```python
from build123d import *

# Parameters (mm, degrees)
F1_DEPTH = 150
F2_SIZE  = 20


with BuildPart() as f1:
    # F0 (on Top) → F1 (new body)
    with BuildSketch(Plane.XY):
        with BuildLine():
            ThreePointArc((40, 13), (36.485281, 21.485281), (28, 25))
            Line((28, 25), (5, 25))
            Line((5, 25), (5, 15))
            Line((5, 15), (-5, 15))
            Line((-5, 15), (-5, 25))
            Line((-5, 25), (-40, 25))
            Line((-40, 25), (-40, -13))
            ThreePointArc((-40, -13), (-36.485281, -21.485281), (-28, -25))
            Line((-28, -25), (-5, -25))
            Line((-5, -25), (-5, -15))
            Line((-5, -15), (5, -15))
            Line((5, -15), (5, -25))
            Line((5, -25), (40, -25))
            Line((40, -25), (40, 13))
        make_face()
        with BuildLine():
            ThreePointArc((-18.122446, 8.968033), (-23.391993, 14.619996), (-16.00245, 12.360026))
            Line((-16.00245, 12.360026), (-3.737005, 4.694123))
            ThreePointArc((-3.737005, 4.694123), (3.179994, 5.08799), (5.857001, -1.30213))
            Line((5.857001, -1.30213), (18.122446, -8.968033))
            ThreePointArc((18.122446, -8.968033), (23.391993, -14.619996), (16.00245, -12.360026))
            Line((16.00245, -12.360026), (3.737005, -4.694123))
            ThreePointArc((3.737005, -4.694123), (-3.179994, -5.08799), (-5.857001, 1.30213))
            Line((-5.857001, 1.30213), (-18.122446, 8.968033))
        make_face(mode=Mode.SUBTRACT)
    extrude(amount=F1_DEPTH)

    # F2
    f2_edges = [f1.edges().sort_by_distance(p)[0] for p in [
        (-40, 25, 75),
        (40, -25, 75),
    ]]
    chamfer(f2_edges, length=F2_SIZE)


solid = f1.part
```
Source: CAD feature listing. Evaluate the final solid. Frame: model axes, mm. A direction names the side the tool comes from. Round coordinates to 2 decimals unless told otherwise and drop trailing zeros. Loops run counter-clockwise (first coordinate to the right, second up) from the corner with the lowest first, then second, coordinate; pieces in that order, holes last. Notation, with made-up numbers: M 21.5,89 L 79.5,89 A25 ccw 79.5,112 Z; hole C 44.25,57 d9. An arc over 180 degrees is marked long. Use a Markdown table: item, result. Add a question column.
1. Cut plane C-C, the plane y = -20.5. Output: boundary loops of the cut face in (x, z).
2. Cut plane A-A, the plane y = -3. Output: boundary loops of the cut face in (x, z).
3. Cut plane D-D, the plane x = 31. Output: boundary loops of the cut face in (y, z), and give its area (3 significant figures).
4. Contact query for flat-ended pins moving along their axis: pin 1 (5 mm diameter, centred on y = -18.5, z = 96, fed in from -X); pin 2 (3 mm diameter, centred on x = -2, z = 43.5, fed in from +Y); pin 3 (4 mm diameter, centred on y = -19.5, z = 128, fed in from -X). Output: stop coordinate, or through.
5. Ray query, line 1 along Y through (x, z) = (20, 117); line 2 along Y through (x, z) = (-20, 97.5); line 3 along X through (y, z) = (5, 141). Return the intervals inside material, ascending. Write a range as [from, to].
6. Pull-direction query (Y, two-part tool) for faces 1 (the cylindrical face through (3.092, 5.142, 73.95)), 2 (the flat face through (40, 4, 74)), 3 (the flat face through (-30, 15, 74)); classes: +Y half, -Y half, draft (parallel to the pull), parting line (faces both ways), or undercut.
7. Set-up query: faces 4 (the flat face through (-5, -20, 74)), 5 (the flat face through (30, -15, 74)), 6 (the flat face through (9.956, -8.581, 73.95)), 7 (the flat face through (5, 20, 74)). Return all of +Z, -Z, +X, -X, +Y, -Y with unobstructed straight access to the full face (end or side cutting, diameter ignored); none if empty.
8. Cut plane B-B, the plane z = 61. Output: boundary loops of the cut face in (x, y), and give its area (3 significant figures).
Solution:
| question | item | result |
|---|---|---|
| 1 | outline | M -37.37,0 L -5,0 L -5,150 L -37.37,150 Z; M 5,0 L 24.5,0 L 24.5,150 L 5,150 Z |
| 2 | outline | M -40,0 L -5.2,0 L -5.2,150 L -40,150 Z; M 8.57,0 L 40,0 L 40,150 L 8.57,150 Z |
| 3 | outline | M -14,0 L 24.62,0 L 24.62,150 L -14,150 Z |
| 3 | area | 5,790 mm2 |
| 4 | pin 1 | stops at x = -39.62 |
| 4 | pin 2 | stops at y = 15 |
| 4 | pin 3 | stops at x = -39.12 |
| 5 | line 1 | y = [-25, -16.5], [-8.5, 25] |
| 5 | line 2 | y = [-25, 8.5], [16.5, 25] |
| 5 | line 3 | x = [-40, -11.77], [-4.23, -3.32], [3.32, 40] |
| 6 | face 1 | undercut |
| 6 | face 2 | draft |
| 6 | face 3 | +Y half |
| 7 | face 4 | +Z, -Z, -Y |
| 7 | face 5 | +Z, -Z, +X, -Y |
| 7 | face 6 | +Z, -Z |
| 7 | face 7 | +Z, -Z, +Y |
| 8 | outline | M -40,-13 A12 ccw -28,-25 L -5,-25 L -5,-15 L 5,-15 L 5,-25 L 20,-25 L 40,-5 L 40,13 A12 ccw 28,25 L 5,25 L 5,15 L -5,15 L -5,25 L -20,25 L -40,5 Z; hole M -18.12,8.97 L -5.86,1.3 A6 ccw 3.74,-4.69 L 16,-12.36 A4 ccw long 18.12,-8.97 L 5.86,-1.3 A6 ccw -3.74,4.69 L -16,12.36 A4 ccw long Z |
| 8 | area | 3,010 mm2 |
